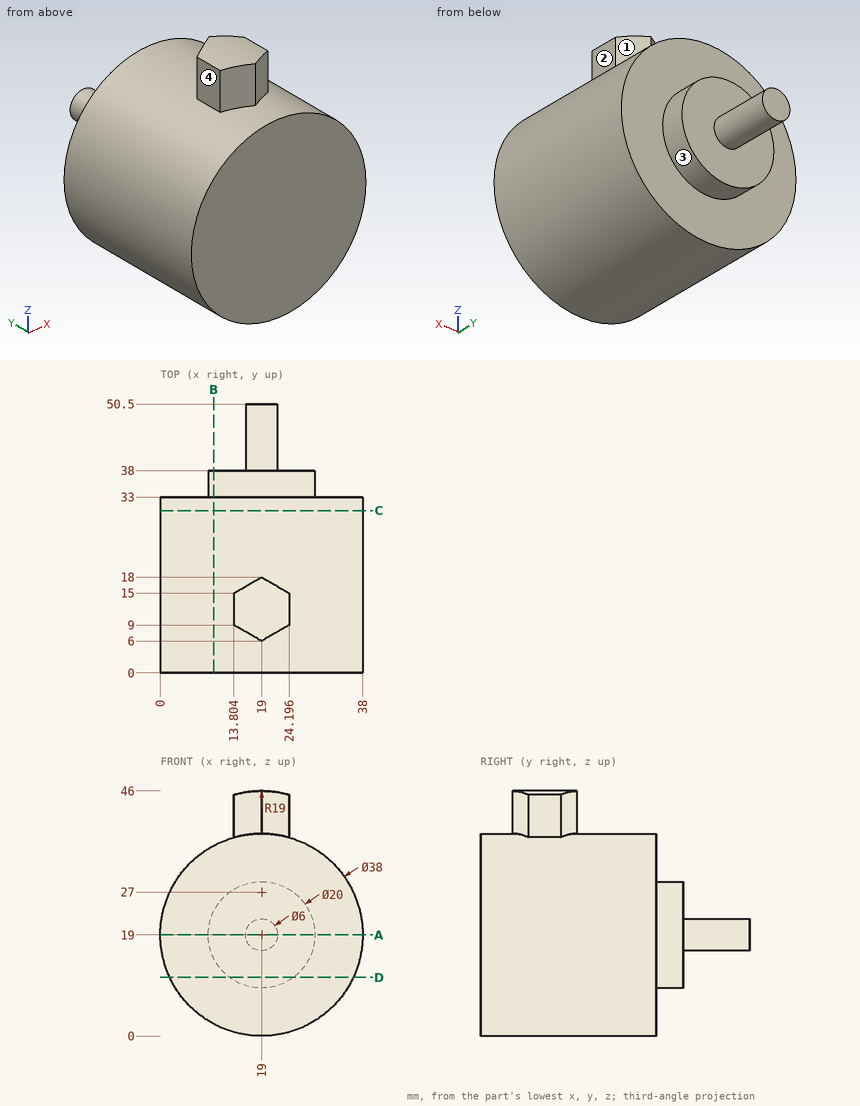
Here's the drawing with two shaded views (mm, measured from the low corner). I have some questions. A direction names the side the tool comes from. Round coordinates to 2 decimals unless told otherwise and drop trailing zeros. Loops run counter-clockwise (first coordinate to the right, second up) from the corner with the lowest first, then second, coordinate; pieces in that order, holes last. Notation, with made-up numbers: M 18.25,-11 L 45.25,-11 A27 ccw 45.25,26 Z; hole C 76,-34 d5. An arc over 180 degrees is marked long. Answer as a JSON object with one key per item and string values. Group by question number.
Q1. Please list where these lines run through material, in increasing order: L1, parallel to Y at x = 23, z = 16.5; L2, parallel to Y at x = 9.5, z = 23; L3, parallel to X at y = 14.5, z = 39.
Q2. On a 3-axis mill with a long thin cutter (end or side, diameter ignored), from which of +Z, -Z, +X, -X, +Y, -Y can I reach the whole of each face in a straight line? I mean the marked faces 1, 2, 3 and 4. Say none if no direction works.
Q3. Will these pins go through, and if not, where does the flat tip stop? pin 1 (1.8 mm diameter, centred on y = 11.5, z = 40.5, fed in from +X); pin 2 (3 mm diameter, centred on x = 31, y = 14.5, fed in from -Z) (1 decimal); pin 3 (6 mm diameter, centred on x = 11, z = 25, fed in from +Y).
Q4. Imagine slicing it at D-D, the plane z = 11. Please give me the cut outline in (x, y), then the cut area to 3 significant figures.
Q5. Imagine slicing it at B-B, the plane x = 10. Please give me the cut outline in (y, z), then the cut area to 3 significant figures.
Q6. Imagine slicing it at A-A, the plane z = 19. Please give me the cut outline in (x, y), then the cut area to 3 significant figures.
Q7. Imagine slicing it at C-C, the plane y = 30.5. Please give me the cut outline in (x, z).
Findings:
{
 "1": {"L1": "y = 0 to 38", "L2": "y = 0 to 33", "L3": "x = 13.8 to 24.2"},
 "2": {"face 1": "+Z, +X, +Y", "face 2": "+Z, +X, +Y, -Y", "face 3": "+Y", "face 4": "+Z, -X, +Y, -Y"},
 "3": {"pin 1": "stops at x = 24.2", "pin 2": "stops at z = 3.2", "pin 3": "stops at y = 38"},
 "4": {"outline": "M 1.77,0 L 36.23,0 L 36.23,33 L 25,33 L 25,38 L 13,38 L 13,33 L 1.77,33 Z", "area": "1,200 mm2"},
 "5": {"outline": "M 0,2.27 L 33,2.27 L 33,14.64 L 38,14.64 L 38,23.36 L 33,23.36 L 33,35.73 L 0,35.73 Z", "area": "1,150 mm2"},
 "6": {"outline": "M 0,0 L 38,0 L 38,33 L 29,33 L 29,38 L 22,38 L 22,50.5 L 16,50.5 L 16,38 L 9,38 L 9,33 L 0,33 Z", "area": "1,430 mm2"},
 "7": {"outline": "C 19,19 d38"}
}
